```python
from build123d import *

# Parameters (mm, degrees)
CROQUIS1_W              = 5
CROQUIS1_H              = 10
CROQUIS1_W_2            = 10
CROQUIS1_H_2            = 5
SALIENTE_EXTRUIR1_DEPTH = 5
CORTAR_EXTRUIR7_DEPTH   = 151
CROQUIS8_W              = 4
CROQUIS8_H              = 5
CROQUIS8_W_2            = 5
CROQUIS8_H_2            = 7.5
CROQUIS8_W_3            = 7
CORTAR_EXTRUIR12_DEPTH  = 10


with BuildPart() as part:
    # Croquis1 → Saliente-Extruir1 (new body)
    with BuildSketch(Plane.XY):
        Polygon((0, 0), (10, 0), (10, 5), (20, 5), (20, 0), (30, 0), (30, 5), (35, 5), (35, 95), (115, 95), (115, 5), (117.5, 5), (120, 5), (120, 0), (130, 0), (130, 5), (140, 5), (140, 0), (150, 0), (150, 15), (145, 15), (145, 25), (150, 25), (150, 35), (145, 35), (145, 45), (150, 45), (150, 55), (145, 55), (145, 65), (150, 65), (150, 75), (145, 75), (145, 85), (150, 85), (150, 95), (145, 95), (145, 105), (150, 105), (150, 115), (145, 115), (145, 125), (150, 125), (150, 135), (145, 135), (145, 145), (150, 145), (150, 155), (145, 155), (145, 165), (150, 165), (150, 175), (145, 175), (145, 185), (150, 185), (150, 200), (0, 200), (0, 185), (5, 185), (5, 175), (0, 175), (0, 165), (5, 165), (5, 155), (0, 155), (0, 145), (5, 145), (5, 135), (0, 135), (0, 125), (5, 125), (5, 115), (0, 115), (0, 105), (5, 105), (5, 95), (0, 95), (0, 85), (5, 85), (5, 75), (0, 75), (0, 65), (5, 65), (5, 55), (0, 55), (0, 45), (5, 45), (5, 35), (0, 35), (0, 25), (5, 25), (5, 15), (0, 15), align=None)
        with Locations((28.99995, 20)):
            Rectangle(CROQUIS1_W, CROQUIS1_H, mode=Mode.SUBTRACT)
        with Locations((28.99995, 40)):
            Rectangle(CROQUIS1_W, CROQUIS1_H, mode=Mode.SUBTRACT)
        with Locations((28.99995, 60)):
            Rectangle(CROQUIS1_W, CROQUIS1_H, mode=Mode.SUBTRACT)
        with Locations((28.99995, 80)):
            Rectangle(CROQUIS1_W, CROQUIS1_H, mode=Mode.SUBTRACT)
        with Locations((28.99995, 100)):
            Rectangle(CROQUIS1_W, CROQUIS1_H, mode=Mode.SUBTRACT)
        with Locations((121.00005, 20)):
            Rectangle(CROQUIS1_W, CROQUIS1_H, mode=Mode.SUBTRACT)
        with Locations((121.00005, 40)):
            Rectangle(CROQUIS1_W, CROQUIS1_H, mode=Mode.SUBTRACT)
        with Locations((121.0005, 60)):
            Rectangle(CROQUIS1_W, CROQUIS1_H, mode=Mode.SUBTRACT)
        with Locations((121.00005, 80)):
            Rectangle(CROQUIS1_W, CROQUIS1_H, mode=Mode.SUBTRACT)
        with Locations((121.00005, 100)):
            Rectangle(CROQUIS1_W, CROQUIS1_H, mode=Mode.SUBTRACT)
        with Locations((28.99995, 120)):
            Rectangle(CROQUIS1_W, CROQUIS1_H, mode=Mode.SUBTRACT)
        with Locations((28.99995, 140)):
            Rectangle(CROQUIS1_W, CROQUIS1_H, mode=Mode.SUBTRACT)
        with Locations((14.25, 152.5)):
            Rectangle(CROQUIS1_W_2, CROQUIS1_H_2, mode=Mode.SUBTRACT)
        with Locations((28.99995, 160)):
            Rectangle(CROQUIS1_W, CROQUIS1_H, mode=Mode.SUBTRACT)
        with Locations((45, 152.5)):
            Rectangle(CROQUIS1_W_2, CROQUIS1_H_2, mode=Mode.SUBTRACT)
        with Locations((65, 152.5)):
            Rectangle(CROQUIS1_W_2, CROQUIS1_H_2, mode=Mode.SUBTRACT)
        with Locations((121.00005, 120)):
            Rectangle(CROQUIS1_W, CROQUIS1_H, mode=Mode.SUBTRACT)
        with Locations((121.00005, 140)):
            Rectangle(CROQUIS1_W, CROQUIS1_H, mode=Mode.SUBTRACT)
        with Locations((85, 152.5)):
            Rectangle(CROQUIS1_W_2, CROQUIS1_H_2, mode=Mode.SUBTRACT)
        with Locations((105, 152.5)):
            Rectangle(CROQUIS1_W_2, CROQUIS1_H_2, mode=Mode.SUBTRACT)
        with Locations((121.00005, 160)):
            Rectangle(CROQUIS1_W, CROQUIS1_H, mode=Mode.SUBTRACT)
    extrude(amount=SALIENTE_EXTRUIR1_DEPTH)

    # Croquis7 → Cortar-Extruir7 (cut, through all)
    with BuildSketch(Plane.ZY):
        Polygon((0, 200), (5.317351356, 198.600697011), (5, 200), align=None)
    extrude(amount=-CORTAR_EXTRUIR7_DEPTH, mode=Mode.SUBTRACT)

    # Croquis8 → Cortar-Extruir12 (cut)
    with BuildSketch(Plane.XY.offset(5)):
        with Locations((129.70005, 90.5)):
            Rectangle(CROQUIS8_W, CROQUIS8_H)
        with Locations((134.20005, 83.75)):
            Rectangle(CROQUIS8_W_2, CROQUIS8_H_2)
        with Locations((138.70005, 90.5)):
            Rectangle(CROQUIS8_W, CROQUIS8_H)
        with Locations((141.5, 98.875)):
            Rectangle(CROQUIS8_W_3, CROQUIS8_H)
    extrude(amount=-CORTAR_EXTRUIR12_DEPTH, mode=Mode.SUBTRACT)


solid = part.part
```
The model under review builds one solid part; all positions refer to its coordinate system, in mm. A direction names the side the tool comes from. Coordinates: 2 decimals unless noted, no trailing zeros. Write each loop counter-clockwise with the first axis right and the second up, starting at its lowest first coordinate (ties: lowest second). Pieces come first, ordered by that corner, then holes.
1) To check wall thickness, follow probe 1 along X at (y, z) = (153.5, 4); probe 2 along X at (y, z) = (163, 1.35); probe 3 along X at (y, z) = (100, 1.2). State the ranges of each line that lie inside material, in increasing order.
2) We need section A-A on y = 20.5. State the section outline as (x, z) points, then the cut area to 3 significant figures.
3) Machinability: for faces 1 (the face through (5, 40, 2)), 2 (the face through (31.5, 60, 2)), 3 (the face through (145, 180, 2)), 4 (the face through (120, 3, 2)), which of the approach directions +Z, -Z, +X, -X, +Y, -Y give a long, thin tool a straight path to every point of the face, cutting with its end or side? Answer none if there is none.
4) We need section B-B on x = 43. State the section outline as (y, z) points.
5) We need section D-D on x = 97.5. State the section outline as (y, z) points, then the cut area to 3 significant figures.
6) We need section C-C on y = 67.5. State the section outline as (x, z) points.
7) Clearance check with flat-ended pins moving along their axes: pin 1 Ø2 at (x, z) = (133, 3) entering from -Y; pin 2 Ø1.1 at (y, z) = (103.5, 1.5) entering from +X; pin 3 Ø1.5 at (x, z) = (147, 3) entering from +Y. State where each tip first meets the part, or that it passes through.
8) The part is to be moulded in two halves that separate along X. For faces 5 (the face through (148, 175, 2)), 6 (the face through (29, 135, 2)), 7 (the face through (0, 150, 2)), say which applies: pulls with the +X half, pulls with the -X half, needs draft (parallel to the pull), parting line crosses it, or undercut.
Answer list:
1. probe 1: x = 0 to 9.25, 19.25 to 40, 50 to 60, 70 to 80, 90 to 100, 110 to 150
1. probe 2: x = 5 to 26.5, 31.5 to 118.5, 123.5 to 145
1. probe 3: x = 5 to 26.5, 31.5 to 118.5, 123.5 to 138
2. outline: (5, 0) - (26.5, 0) - (26.5, 5) - (5, 5) - close; (31.5, 0) - (35, 0) - (35, 5) - (31.5, 5) - close; (115, 0) - (118.5, 0) - (118.5, 5) - (115, 5) - close; (123.5, 0) - (145, 0) - (145, 5) - (123.5, 5) - close
2. area: 250 mm2
3. face 1: +Z, -Z, -X
3. face 2: +Z, -Z
3. face 3: +Z, -Z, +X
3. face 4: +Z, -Z, -Y
4. outline: (95, 0) - (150, 0) - (150, 5) - (95, 5) - close; (155, 0) - (200, 0) - (198.68, 5) - (155, 5) - close
5. outline: (95, 0) - (200, 0) - (198.68, 5) - (95, 5) - close
5. area: 522 mm2
6. outline: (0, 0) - (35, 0) - (35, 5) - (0, 5) - close; (115, 0) - (150, 0) - (150, 5) - (115, 5) - close
7. pin 1: stops at y = 5
7. pin 2: stops at x = 145
7. pin 3: stops at y = 199.41
8. face 5: needs draft
8. face 6: undercut
8. face 7: pulls with the -X half
